```python
from build123d import *

# Parameters (mm, degrees)
SKETCH029_R     = 3.5
SKETCH029_R_2   = 2.45
PAD016_DEPTH    = 5
PAD017_DEPTH    = 3
SKETCH032_R     = 21.114958
POCKET017_DEPTH = 1
SKETCH033_W     = 11.558153
SKETCH033_H     = 2.526367
SKETCH033_W_2   = 11.494995
PAD018_DEPTH    = 1.8
SKETCH034_W     = 1.3
SKETCH034_H     = 2.5
POCKET018_DEPTH = 1
FILLET002_R     = 0.4


with BuildPart() as part:
    # Sketch029 (on DatumPlane) → Pad016 (new body)
    with BuildSketch(Plane(origin=(-141.5, 0, 0), x_dir=(0, -1, 0), z_dir=(-1, 0, 0))):
        with BuildLine():
            Line((-60.710533, -22.509186), (-60.710533, -87.509186))
            Line((-60.710533, -87.509186), (0, -76.804281))
            ThreePointArc((0, -76.804281), (18.288256, -55.009186), (0, -33.214091))
            Line((-60.710533, -22.509186), (0, -33.214091))
        make_face()
        with Locations((5.001089, -55.009186)):
            Circle(SKETCH029_R, mode=Mode.SUBTRACT)
        with Locations((-39.998911, -55.009186)):
            Circle(SKETCH029_R_2, mode=Mode.SUBTRACT)
    extrude(amount=-PAD016_DEPTH)

    # Sketch031 (on Face7 of Pad016) → Pad017 (join)
    with BuildSketch(Plane(origin=(-141.5, 0, 0), x_dir=(0, -1, 0), z_dir=(-1, 0, 0))):
        with BuildLine():
            Line((0, -76.804281), (-40.654194, -66.047978))
            ThreePointArc((-40.691972, -43.826584), (-47.888023, -54.949547), (-40.654194, -66.047978))
            Line((-40.691972, -43.826584), (0, -33.214091))
            Line((0, -33.214091), (-60.710533, -22.509186))
            Line((-60.710533, -22.509186), (-60.710533, -87.509186))
            Line((-60.710533, -87.509186), (0, -76.804281))
        make_face()
    extrude(amount=PAD017_DEPTH)

    # Sketch032 (on Face12 of Pad017) → Pocket017 (cut)
    with BuildSketch(Plane(origin=(-141.5, 0, 0), x_dir=(0, -1, 0), z_dir=(-1, 0, 0))):
        with Locations((5.001089, -55.009186)):
            Circle(SKETCH032_R)
    extrude(amount=-POCKET017_DEPTH, mode=Mode.SUBTRACT)

    # Sketch033 (on Face1 of Pocket017) → Pad018 (join)
    with BuildSketch(Plane(origin=(-155, 60.710533, 0), x_dir=(0, 0, -1), z_dir=(0, 1, 0))):
        with Locations((33.659026, -15.995544)):
            Rectangle(SKETCH033_W, SKETCH033_H)
        with Locations((76.070472, -15.995544)):
            Rectangle(SKETCH033_W_2, SKETCH033_H)
    extrude(amount=PAD018_DEPTH)

    # Sketch034 (on Face24 of Pad018) → Pocket018 (cut)
    with BuildSketch(Plane(origin=(-140.5, 0, 0), x_dir=(0, -1, 0), z_dir=(-1, 0, 0))):
        with Locations((-2.756497, -55.009186)):
            Rectangle(SKETCH034_W, SKETCH034_H)
    extrude(amount=-POCKET018_DEPTH, mode=Mode.SUBTRACT)

    # Fillet002
    fillet002_edges = [part.edges().sort_by_distance(p)[0] for p in [
        (-140.267639, 62.510533, -76.070473),
        (-139.004456, 62.510533, -81.81797),
        (-137.741272, 62.510533, -76.070473),
        (-139.004456, 62.510533, -70.322975),
        (-140.267639, 62.510533, -33.659027),
        (-139.004456, 62.510533, -39.438103),
        (-137.741272, 62.510533, -33.659027),
        (-139.004456, 62.510533, -27.87995),
    ]]
    fillet(fillet002_edges, radius=FILLET002_R)


solid = part.part
```
Geometry check sheet. Reference: the model listing, model coordinates, mm. A direction names the side the tool comes from. Coordinates: 2 decimals unless noted, no trailing zeros. Write each loop counter-clockwise with the first axis right and the second up, starting at its lowest first coordinate (ties: lowest second). Pieces come first, ordered by that corner, then holes. Notation, with made-up numbers: M 67.5,4.25 L 116.5,4.25 A13 ccw 116.5,20.25 Z; hole C 23.5,45.5 d4. An arc over 180 degrees is marked long. One line per item, written item: value. Start each with the question number.
(1) Sectioned sample at D-D, the plane y = 36. Enter the section's corners in (x, z).
(2) Tool access check on faces 4 (the face through (-142.979, 20.631, -38.595)), 5 (the face through (-136.5, 31, -55)). Record the directions out of +Z, -Z, +X, -X, +Y, -Y that give a thin tool (end or side, any length) a straight path to the whole face; none if there is none.
(3) Sectioned sample at C-C, the plane z = -80.5. Enter the section's corners in (x, y).
(4) Sectioned sample at A-A, the plane y = 5.5. Enter the section's corners in (x, z).
(5) Depth check by flat-ended pin: pin 1 (0.5 mm diameter, centred on x = -140, y = 3, fed in from +Z); pin 2 (4 mm diameter, centred on x = -142.5, y = 7, fed in from -Z); pin 3 (1.5 mm diameter, centred on y = 61.5, z = -75.5, fed in from -X); pin 4 (5.5 mm diameter, centred on y = 40, z = -55.01, fed in from +X). Enter the tip coordinate at first touch or a pass-through.
(6) Sectioned sample at B-B, the plane z = -72. Enter the section's corners in (x, y) (3 decimals), and give its area (3 significant figures).
(7) Release check for a two-part mould opening along Z. For faces 1 (the face through (-138.479, -18.284, -55.442)), 2 (the face through (-139, 62.511, -34)), 3 (the face through (-138.528, -2.421, -52.644)) record: released by +Z, released by -Z, zero draft, split by the parting line, or undercut.
(8) Scan lines: line 1 along X through (y, z) = (-8, -49); line 2 along Z through (x, y) = (-143.75, 33.5); line 3 along X through (y, z) = (37.5, -60). Record each from-to range of solid material in increasing order. Write a range as [from, to].
Filled sheet:
1. outline: M -144.5,-83.15 L -136.5,-83.15 L -136.5,-26.87 L -144.5,-26.87 L -144.5,-42.6 L -141.5,-42.6 L -141.5,-67.28 L -144.5,-67.28 Z
2. face 4: -X, -Y
2. face 5: +Z, -Z, +X, +Y, -Y
3. outline: M -144.5,20.96 L -136.5,20.96 L -136.5,60.71 L -137.74,60.71 L -137.74,62.11 A0.4 ccw -138.14,62.51 L -139.87,62.51 A0.4 ccw -140.27,62.11 L -140.27,60.71 L -144.5,60.71 Z
4. outline: M -144.5,-77.77 L -136.5,-77.77 L -136.5,-32.24 L -144.5,-32.24 L -144.5,-34.65 L -141.5,-34.65 L -141.5,-36.69 L -140.5,-36.69 L -140.5,-73.33 L -141.5,-73.33 L -141.5,-75.35 L -144.5,-75.35 Z
5. pin 1: z = -32.64
5. pin 2: z = -78.39
5. pin 3: x = -140.27
5. pin 4: x = -136.5
6. outline: M -144.5,18.158 L -141.5,18.158 L -141.5,7.535 L -140.5,7.535 L -140.5,-10.338 L -136.5,-10.338 L -136.5,60.711 L -137.741,60.711 L -137.741,62.111 A0.4 ccw -138.141,62.511 L -139.868,62.511 A0.4 ccw -140.268,62.111 L -140.268,60.711 L -144.5,60.711 Z
6. area: 470 mm²
7. face 1: split by the parting line
7. face 2: zero draft
7. face 3: undercut
8. line 1: [-140.5, -136.5]
8. line 2: [-82.71, -67.94], [-41.95, -27.31]
8. line 3: [-141.5, -136.5]
